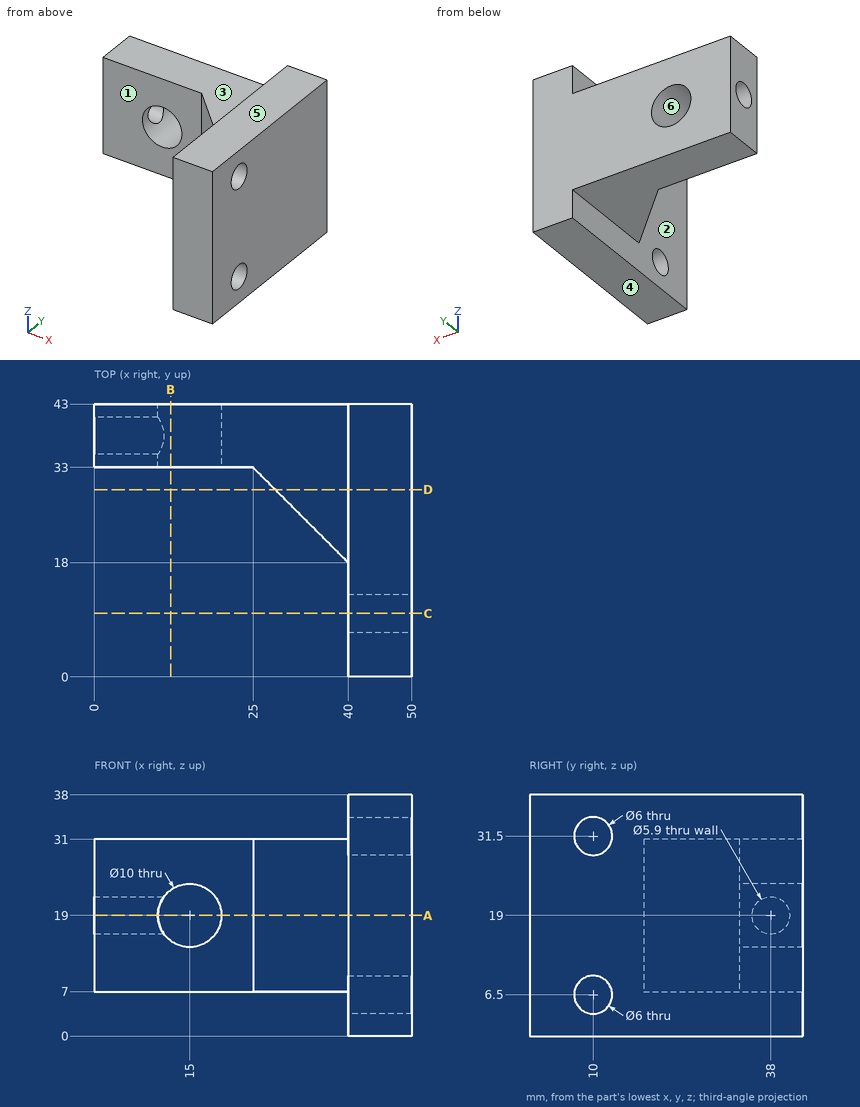
Check sheet for the drawn part. Datum: minimum x, y, z corner. Units: mm. A direction names the side the tool comes from. Round coordinates to 2 decimals unless told otherwise and drop trailing zeros. Loops run counter-clockwise (first coordinate to the right, second up) from the corner with the lowest first, then second, coordinate; pieces in that order, holes last. Notation, with made-up numbers: M 50,21.5 L 67,21.5 A21 ccw 67,29.5 Z; hole C 38,77.25 d9. An arc over 180 degrees is marked long. Write each question's results on one line, items separated by ' | '.
1) Access from +Z, -Z, +X, -X, +Y, -Y to the whole of each face (thin tool, end or side, straight path). Record for the marked faces 1, 2 and 3.
Checks:
face 1: +Z, -Z, -X, -Y | face 2: -X, -Y | face 3: +Z, -X, +Y, -Y
2) Section check B-B on x = 12. Record the boundary of the cut face in (y, z), then the cut area to 3 significant figures.
Checks:
outline: M 33,7 L 43,7 L 43,15 L 33,15 Z; M 33,23 L 43,23 L 43,31 L 33,31 Z | area: 160 mm2
3) Gauge pin test, flat ends, axial feed: P1, Ø2, axis at x = 37.5, y = 28.5, coming from the +Z side; P2, Ø12, axis at x = 22.5, z = 9, coming from the -Y side; P3, Ø5, axis at x = 6, z = 17, coming from the -Y side. Record the tip position at first contact, or that the pin passes through.
Checks:
P1: stops at z = 31 | P2: stops at y = 29.5 | P3: stops at y = 33
4) Section check A-A on z = 19. Record the boundary of the cut face in (x, y), then the cut area to 4 significant figures.
Checks:
outline: M 0,33 L 10,33 L 10,35.05 L 0,35.05 Z; M 0,40.95 L 10,40.95 L 10,43 L 0,43 Z; M 20,33 L 25,33 L 40,18 L 40,0 L 50,0 L 50,43 L 20,43 Z | area: 783.5 mm2
5) Mould release check, pull along Z, two halves, no side actions. Record for the marked faces 4, 5 and 6: released by +Z, released by -Z, zero draft, split by the parting line, or undercut.
Checks:
face 4: released by -Z | face 5: released by +Z | face 6: undercut
6) Section check C-C on y = 10. Record the boundary of the cut face in (x, z).
Checks:
outline: M 40,0 L 50,0 L 50,3.5 L 40,3.5 Z; M 40,9.5 L 50,9.5 L 50,28.5 L 40,28.5 Z; M 40,34.5 L 50,34.5 L 50,38 L 40,38 Z
7) Scan lines: L1, parallel to Z at x = 15, y = 35.75; L2, parallel to Y at x = 8, z = 19; L3, parallel to Z at x = 5.75, y = 38. Record each from-to range of solid material in increasing order. Write a range as from..to.
Checks:
L1: z = 7..14, 24..31 | L2: y = 33..35.05, 40.95..43 | L3: z = 7..16.05, 21.95..31
8) Section check D-D on y = 29.5. Record the boundary of the cut face in (x, z), then the cut area to 3 significant figures.
Checks:
outline: M 28.5,7 L 40,7 L 40,0 L 50,0 L 50,38 L 40,38 L 40,31 L 28.5,31 Z | area: 656 mm2
